Part model, mm, in its own coordinate system. A direction names the side the tool comes from. Round coordinates to 2 decimals unless told otherwise and drop trailing zeros. Write each loop counter-clockwise with the first axis right and the second up, starting at its lowest first coordinate (ties: lowest second). Pieces come first, ordered by that corner, then holes. Notation, with made-up numbers: M -34,40 L -30,40 A20 ccw -30,56 Z; hole C 26,67.25 d3. An arc over 180 degrees is marked long. Use a Markdown table: item, result. Add a question column.
1) Slice it at D-D on y = -12.25. Write the cut outline in (x, z), plus the area to 3 significant figures.
2) Slice it at A-A on x = 0. Write the cut outline in (y, z), plus the area to 3 significant figures.
3) Slice it at C-C on z = 15.5. Write the cut outline in (x, y), plus the area to 3 significant figures.
4) Wall check: probe 1 along Z at (x, y) = (0, -3.6); probe 2 along Y at (x, z) = (-18, 8.5); probe 3 along Z at (x, y) = (8, -5.75). Give the ranges that are in metal, low to high.
5) Which spindle directions (+Z, -Z, +X, -X, +Y, -Y) get a long thin tool onto all of the face, cutting with end or side? Do faces 1 (the face through (25.35, -0.68, -13.1)), 2 (the face through (18.11, -1.48, -16.23)), 3 (the face through (1.4, -1.35, 25.8)). Say none if no direction does.
6) Two-plate mould, pull along Z, no slides. Class faces 4 (the face through (-0.234, -0.684, 29.075)), 5 (the face through (-18.19, -1.479, -16.276)), 6 (the face through (-5, -1, 24)): released by +Z, released by -Z, zero draft, split by the parting line, or undercut.
7) Drop flat-ended pins along their axis: P1, Ø0.9, axis at y = -1.5, z = 25.5, coming from the -X side; P2, Ø3, axis at x = 1.5, y = -5.5, coming from the -Z side; P3, Ø0.9, axis at y = -1.5, z = 23, coming from the +X side; P4, Ø3.5, axis at x = 2, z = 2, coming from the -Y side. Give the stop position or say it passes through.
8) Slice it at B-B on z = 0. Write the cut outline in (x, y).
```python
from build123d import *

# Parameters (mm, degrees)
F1_DEPTH  = 3
F2_R      = 19.0263418025
F2_R_2    = 16.5382084955
F3_DEPTH  = 11
F4_R      = 5
F5_DEPTH  = 3.001
F7_R      = 1.8
F8_DEPTH  = 3.001
F6_R      = 6
F6_R_2    = 5
F9_DEPTH  = 1
F10_R     = 3.35
F10_R_2   = 1.8
F11_DEPTH = 1.65
F12_R     = 3.35
F12_R_2   = 1.8
F13_DEPTH = 1.65


with BuildPart() as f1:
    # F0 (on Front) → F1 (new body)
    with BuildSketch(Plane.XZ):
        with BuildLine():
            Line((-5, 27.2899847478), (-5, 20.3960780544))
            ThreePointArc((-5, 20.3960780544), (-18.1865334795, 10.5), (-20.1635217327, -5.8679120083))
            Line((-20.1635217327, -5.8679120083), (-26.1338200605, -9.314865355))
            ThreePointArc((-26.1338200605, -9.314865355), (-27.9639470794, -16.1449923739), (-21.1338200605, -17.9751193928))
            Line((-21.1338200605, -17.9751193928), (-15.1635217327, -14.5281660461))
            ThreePointArc((-15.1635217327, -14.5281660461), (0, -21), (15.1635217327, -14.5281660461))
            Line((15.1635217327, -14.5281660461), (21.1338200605, -17.9751193928))
            ThreePointArc((21.1338200605, -17.9751193928), (27.9639470794, -16.1449923739), (26.1338200605, -9.314865355))
            Line((26.1338200605, -9.314865355), (20.1635217327, -5.8679120083))
            ThreePointArc((20.1635217327, -5.8679120083), (18.1865334795, 10.5), (5, 20.3960780544))
            Line((5, 20.3960780544), (5, 27.2899847478))
            ThreePointArc((5, 27.2899847478), (0, 32.2899847478), (-5, 27.2899847478))
        make_face()
    extrude(amount=F1_DEPTH)

    # F2 (on face) → F3 (join)
    with BuildSketch(Plane.XZ.offset(3)):
        Circle(F2_R)
        Circle(F2_R_2, mode=Mode.SUBTRACT)
    extrude(amount=F3_DEPTH)

    # F4 (on face) → F5 (cut, through all)
    with BuildSketch(Plane.XZ.offset(3)):
        Circle(F4_R)
    extrude(amount=-F5_DEPTH, mode=Mode.SUBTRACT)

    # F7 (on face) → F8 (cut, through all)
    with BuildSketch(Plane.XZ.offset(3)):
        with Locations((-23.6338200605, -13.6449923739)):
            Circle(F7_R)
        with Locations((23.6338200605, -13.6449923739)):
            Circle(F7_R)
        with Locations((0, 27.2899847478)):
            Circle(F7_R)
    extrude(amount=-F8_DEPTH, mode=Mode.SUBTRACT)

    # F6 (on face) → F9 (join)
    with BuildSketch(Plane.XZ.offset(3)):
        Circle(F6_R)
        Circle(F6_R_2, mode=Mode.SUBTRACT)
    extrude(amount=F9_DEPTH)

    # F10 (on face) → F11 (cut)
    with BuildSketch(Plane.XZ.offset(3)):
        with Locations((0, 27.2899847478)):
            Circle(F10_R)
        with Locations((0, 27.2899847478)):
            Circle(F10_R_2, mode=Mode.SUBTRACT)
    extrude(amount=-F11_DEPTH, mode=Mode.SUBTRACT)

    # F12 (on face) → F13 (cut)
    with BuildSketch(Plane.XZ.offset(3)):
        with Locations((23.6338200605, -13.6449923739)):
            Circle(F12_R)
        with Locations((23.6338200605, -13.6449923739)):
            Circle(F12_R_2, mode=Mode.SUBTRACT)
        with Locations((-23.6338200605, -13.6449923739)):
            Circle(F12_R)
        with Locations((-23.6338200605, -13.6449923739)):
            Circle(F12_R_2, mode=Mode.SUBTRACT)
    extrude(amount=-F13_DEPTH, mode=Mode.SUBTRACT)


solid = f1.part
```
Entries:
| question | item | result |
|---|---|---|
| 1 | outline | C 0,0 d38.05; hole C 0,0 d33.08 |
| 1 | area | 278 mm^2 |
| 2 | outline | M -14,-19.03 L -3,-19.03 L -3,-21 L 0,-21 L 0,-5 L -4,-5 L -4,-6 L -3,-6 L -3,-16.54 L -14,-16.54 Z; M -14,16.54 L -3,16.54 L -3,6 L -4,6 L -4,5 L 0,5 L 0,25.49 L -1.35,25.49 L -1.35,23.94 L -3,23.94 L -3,19.03 L -14,19.03 Z; M -3,30.64 L -1.35,30.64 L -1.35,29.09 L 0,29.09 L 0,32.29 L -3,32.29 Z |
| 2 | area | 171 mm^2 |
| 3 | outline | M -14.17,-3 L -11.03,-3 L -11.03,-14 L -5.77,-14 L -5.77,-3 L 5.77,-3 L 5.77,-14 L 11.03,-14 L 11.03,-3 L 14.17,-3 L 14.17,0 L -14.17,0 Z |
| 3 | area | 201 mm^2 |
| 4 | probe 1 | z = -19.03 to -16.54, -6 to -5, 5 to 6, 16.54 to 19.03 |
| 4 | probe 2 | y = -3 to 0 |
| 4 | probe 3 | z = -17.26 to -14.47, 14.47 to 17.26 |
| 5 | face 1 | +Y, -Y |
| 5 | face 2 | -Z, +Y, -Y |
| 5 | face 3 | -Y |
| 6 | face 4 | undercut |
| 6 | face 5 | released by -Z |
| 6 | face 6 | zero draft |
| 7 | P1 | stops at x = -5 |
| 7 | P2 | stops at z = -19.03 |
| 7 | P3 | stops at x = 5 |
| 7 | P4 | passes through |
| 8 | outline | M -21,-3 L -19.03,-3 L -19.03,-14 L -16.54,-14 L -16.54,-3 L -6,-3 L -6,-4 L -5,-4 L -5,0 L -21,0 Z; M 5,-4 L 6,-4 L 6,-3 L 16.54,-3 L 16.54,-14 L 19.03,-14 L 19.03,-3 L 21,-3 L 21,0 L 5,0 Z |
